Solid Edge part; units mm, degrees
sketch "Sketch1" plane through (0, 0, 0) normal (0, -1, 0) x (1, 0, 0)
  line L0 (-36, 0) -> (0, 0)
  line L1 (0, 0) -> (0, 36)
  line L2 (0, 36) -> (4, 36)
  line L3 (4, 36) -> (4, -4)
  line L4 (4, -4) -> (-36, -4)
  line L5 (-36, -4) -> (-36, 0)
extrude "Protrusion1" add sketch "Sketch1" along normal mid plane 350
sketch "Sketch2" plane through (-18, 0, 0) normal (0, 0, 1) x (0, -1, 0)
  circle A0 centre (-155, 8) radius 3
  circle A1 centre (-155, -10) radius 3
  dimension "D1" = 155
  dimension "D2" = 155
extrude "Cutout1" cut sketch "Sketch2" against normal through all
mirror "Mirror1" about plane through (0, 0, 0) normal (0, -1, 0) of "Cutout1"
sketch "Sketch3" plane through (0, 0, 18) normal (-1, 0, 0) x (0, -1, 0)
  line L0 (-22.5, -18) -> (22.5, -18)
  line L1 (22.5, -18) -> (22.5, 18)
  line L2 (22.5, 18) -> (-22.5, 18)
  line L3 (-22.5, 18) -> (-22.5, -18)
  dimension "D1" = 22.5
extrude "Cutout2" cut sketch "Sketch3" against normal through all
properties material "AlSi7Mg"
Verification items for the finished model (mm, model axes). A direction names the side the tool comes from. Round coordinates to 2 decimals unless told otherwise and drop trailing zeros. Order: outer loops, then holes, each group sorted by start corner. A loop starts at its lowest first (then second) coordinate and runs counter-clockwise, first axis right, second up. Notation, with made-up numbers: (24, -10.75) -> (32, -10.75) arc R30 cw to (32, 18.25) -> close; hole circle Ø6 at (10, 51.5). An arc over 180 degrees is marked (long way). Put each result on its own line as item: value. Start each with the question number.
(1) Section check D-D (y = -84). Enter the section's corners in (x, z).
(2) Depth check by flat-ended pin: pin 1 Ø18 at (y, z) = (136.5, 24) entering from -X; pin 2 Ø7 at (x, y) = (-28, 155) entering from +Z. Enter the tip coordinate at first touch or a pass-through.
(3) Tool access check on faces 4 (the face through (0, -98, 18)), 5 (the face through (-10.9, -152.14, -1.97)). Record the directions out of +Z, -Z, +X, -X, +Y, -Y that give a thin tool (end or side, any length) a straight path to the whole face; none if there is none.
(4) Section check A-A (z = 30.5). Enter the section's corners in (x, y).
(5) Draft check along Y on faces 1 (the face through (-9.1, 152.14, -1.97)), 2 (the face through (-7, -175, -0.4)), 3 (the face through (-7, 175, -0.4)). Enter one of: +Y half, -Y half, draft (parallel to the pull), parting line (faces both ways), or undercut.
(6) Section check B-B (x = -10). Enter the section's corners in (y, z), then the cut area to 3 significant figures.
(7) Material ranges on line 1 along X through (y, z) = (-155, -1.1); line 2 along X through (y, z) = (-40.5, 25); line 3 along Z through (x, y) = (-9, -85), recorded low to high.
(8) Section check C-C (y = -155). Enter the section's corners in (x, z), then the cut area to 3 significant figures.
Completed:
1. outline: (-36, -4) -> (4, -4) -> (4, 36) -> (0, 36) -> (0, 0) -> (-36, 0) -> close
2. pin 1: stops at x = 0
2. pin 2: stops at z = 0
3. face 4: +Z, -X, +Y, -Y
3. face 5: +Z, -Z
4. outline: (0, -175) -> (4, -175) -> (4, -22.5) -> (0, -22.5) -> close; (0, 22.5) -> (4, 22.5) -> (4, 175) -> (0, 175) -> close
5. face 1: undercut
5. face 2: -Y half
5. face 3: +Y half
6. outline: (-175, -4) -> (-158, -4) -> (-158, 0) -> (-175, 0) -> close; (-152, -4) -> (152, -4) -> (152, 0) -> (-152, 0) -> close; (158, -4) -> (175, -4) -> (175, 0) -> (158, 0) -> close
6. area: 1,350 mm2
7. line 1: x = -36 to -31, -25 to -13, -7 to 4
7. line 2: x = 0 to 4
7. line 3: z = -4 to 0
8. outline: (-36, -4) -> (-31, -4) -> (-31, 0) -> (-36, 0) -> close; (-25, -4) -> (-13, -4) -> (-13, 0) -> (-25, 0) -> close; (-7, -4) -> (4, -4) -> (4, 36) -> (0, 36) -> (0, 0) -> (-7, 0) -> close
8. area: 256 mm2
